```python
from build123d import *

# Parameters (mm, degrees)
F1_DEPTH = 171.45
F2_R     = 5.5626
F3_DEPTH = 72.8730407724
F4_R     = 3.9751
F5_DEPTH = 76.9722036075


# Not quite as in the source:
# - a feature of the source that left no trace in its solid (it failed there, or was rolled back) is left out


with BuildPart() as f1:
    # F0 (on Top) → F1 (new body)
    with BuildSketch(Plane.XY):
        with BuildLine():
            Line((0, -3.175), (0, 0))
            Line((0, 0), (-28.4702794834, 0))
            ThreePointArc((-28.4702794834, 0), (-30.5376372642, 0.3459570449), (-32.3797298517, 1.3461317146))
            Line((-32.3797298517, 1.3461317146), (-119.8649039531, 69.6970407724))
            Line((-119.8649039531, 69.6970407724), (-121.8196291372, 67.1951066297))
            Line((-121.8196291372, 67.1951066297), (-34.3344550359, -1.1558024281))
            ThreePointArc((-34.3344550359, -1.1558024281), (-31.5713161546, -2.6560644326), (-28.4702794834, -3.175))
            Line((-28.4702794834, -3.175), (0, -3.175))
        make_face()
    extrude(amount=F1_DEPTH)

    # F2 (on face) → F3 (cut, through all)
    with BuildSketch(Plane.XZ.offset(3.175)):
        with Locations((-15.875, 152.4)):
            Circle(F2_R)
        with Locations((-15.875, 38.1)):
            Circle(F2_R)
    extrude(amount=-F3_DEPTH, mode=Mode.SUBTRACT)

    # F4 (on face) → F5 (cut, through all)
    with BuildSketch(Plane(origin=(-13.5748343728, -17.3749956639, 0), x_dir=(0.7880107536, -0.6156614753, 0), z_dir=(-0.6156614753, -0.7880107536, 0))):
        with Locations((-126.2394162429, 81.28)):
            Circle(F4_R)
        with Locations((-40.5144162429, 81.28)):
            Circle(F4_R)
        with Locations((-40.5144162429, 25.4)):
            Circle(F4_R)
        with Locations((-126.2394162429, 25.4)):
            Circle(F4_R)
    extrude(amount=-F5_DEPTH, mode=Mode.SUBTRACT)


solid = f1.part
```
Part model, mm, in its own coordinate system. Coordinates: 2 decimals unless noted, no trailing zeros. Order: outer loops, then holes, each group sorted by start corner. A loop starts at its lowest first (then second) coordinate and runs counter-clockwise, first axis right, second up. Notation, with made-up numbers: (7.5, 86.25) -> (41.5, 86.25) arc R24 cw to (41.5, 122.25) -> close; hole circle Ø8 at (65.25, 72.5). An arc over 180 degrees is marked (long way). Put each result on its own line as item: value. Start each with the question number.
(1) Pin check, flat tips, straight feed: pin 1 Ø2 at (y, z) = (14.5, 120) entering from +X; pin 2 Ø4 at (x, z) = (-44, 82) entering from +Y; pin 3 Ø2 at (y, z) = (23.5, 144.5) entering from +X. Stop position of each tip, or through.
(2) Band-saw the part on D-D (y = 22). Give the cut face in (x, z).
(3) Band-saw the part on B-B (z = 141). Give the cut face in (x, y) (3 decimals), then the cut area to 3 significant figures.
(4) Band-saw the part on A-A (z = 38.1). Give the cut face in (x, y) (3 decimals), then the cut area to 3 significant figures.
(5) Mould opens along Z. For faces 1 (the face through (-14, 0, 85)), 2 (the face through (-66, 25, 171.45)), 3 (the face through (-17.08, -1.61, 146.97)) say: pulls with the +Z half, pulls with the -Z half, needs draft (parallel to the pull), parting line crosses it, or undercut.
(6) Probe line 1 along Y through (x, z) = (-5, 71) (3 decimals); line 2 along Z through (x, y) = (-47, 10); line 3 along X through (y, z) = (-2, 38). List the from-to ranges inside material, lowest first. Write a range as [from, to].
(7) Band-saw the part on C-C (x = -25.5). Give the cut face in (y, z) (3 decimals), then the cut area to 3 significant figures.
Determined:
1. pin 1: stops at x = -47.94
1. pin 2: stops at y = 5.89
1. pin 3: stops at x = -59.46
2. outline: (-63.97, 0) -> (-58.82, 0) -> (-58.82, 171.45) -> (-63.97, 171.45) -> close
3. outline: (-121.82, 67.195) -> (-34.334, -1.156) arc R9.525 ccw to (-28.47, -3.175) -> (0, -3.175) -> (0, 0) -> (-28.47, 0) arc R6.35 cw to (-32.38, 1.346) -> (-119.865, 69.697) -> close
3. area: 460 mm²
4. outline: (-121.82, 67.195) -> (-34.334, -1.156) arc R9.525 ccw to (-28.47, -3.175) -> (-21.438, -3.175) -> (-21.438, 0) -> (-28.47, 0) arc R6.35 cw to (-32.38, 1.346) -> (-119.865, 69.697) -> close; (-10.312, -3.175) -> (0, -3.175) -> (0, 0) -> (-10.312, 0) -> close
4. area: 424 mm²
5. face 1: needs draft
5. face 2: pulls with the +Z half
5. face 3: undercut
6. line 1: y = [-3.175, 0]
6. line 2: z = [0, 22.46], [28.34, 78.34], [84.22, 171.45]
6. line 3: x = [-33.05, -21.44], [-10.31, 0]
7. outline: (-3.175, 0) -> (0, 0) -> (0, 171.45) -> (-3.175, 171.45) -> close
7. area: 544 mm²
